```python
from build123d import *

# Parameters (mm, degrees)
CHAMFER1_SIZE                                  = 1.27
CBORE_FOR_2_SOCKET_HEAD_CAP_SCREW1_D           = 2.7051
CBORE_FOR_2_SOCKET_HEAD_CAP_SCREW1_DEPTH       = 12.7
CBORE_FOR_2_SOCKET_HEAD_CAP_SCREW1_CBORE_D     = 4.7625
CBORE_FOR_2_SOCKET_HEAD_CAP_SCREW1_CBORE_DEPTH = 2.1844
CUT_EXTRUDE1_DEPTH                             = 13.7
SKETCH7_R                                      = 1.27
CUT_EXTRUDE2_DEPTH                             = 13.7


with BuildPart() as part:
    # Sketch1 → Revolve1 (revolve)
    with BuildSketch(Plane.XY):
        Polygon((4, 19.05), (9.525, 19.05), (9.525, 12.7), (19.05, 12.7), (19.05, 0), (4, 0), align=None)
    revolve(axis=Axis((0, 24.600281955, 0), (0, -1, 0)))

    # Chamfer1
    chamfer1_edges = [part.edges().sort_by_distance(p)[0] for p in [
        (-19.05, 12.7, 0),
        (-9.525, 19.05, 0),
        (-4, 19.05, 0),
    ]]
    chamfer(chamfer1_edges, length=CHAMFER1_SIZE)

    # CBORE for #2 Socket Head Cap Screw1
    with Locations(Plane(origin=(0, 12.7, 0), x_dir=(1, 0, 0), z_dir=(0, 1, 0))):
        with Locations((-8.89, -8.89), (8.89, -8.89), (8.89, 8.89), (-8.89, 8.89)):
            CounterBoreHole(CBORE_FOR_2_SOCKET_HEAD_CAP_SCREW1_D / 2, CBORE_FOR_2_SOCKET_HEAD_CAP_SCREW1_CBORE_D / 2, CBORE_FOR_2_SOCKET_HEAD_CAP_SCREW1_CBORE_DEPTH, depth=CBORE_FOR_2_SOCKET_HEAD_CAP_SCREW1_DEPTH)

    # Sketch6 → Cut-Extrude1 (cut, through all)
    with BuildSketch(Plane(origin=(0, 12.7, 0), x_dir=(1, 0, 0), z_dir=(0, 1, 0))):
        with BuildLine():
            Line((12.999999, 1.8415), (18.960785262, 1.8415))
            ThreePointArc((18.960785262, 1.8415), (19.05, 0), (18.960785262, -1.8415))
            Line((18.960785262, -1.8415), (12.999999, -1.8415))
            ThreePointArc((12.999999, -1.8415), (9.9045, 0), (12.999999, 1.8415))
        make_face()
    extrude(amount=-CUT_EXTRUDE1_DEPTH, mode=Mode.SUBTRACT)

    # Sketch7 → Cut-Extrude2 (cut, through all)
    with BuildSketch(Plane(origin=(0, 12.7, 0), x_dir=(1, 0, 0), z_dir=(0, 1, 0))):
        with Locations((-12.7, 0)):
            Circle(SKETCH7_R)
    extrude(amount=-CUT_EXTRUDE2_DEPTH, mode=Mode.SUBTRACT)


solid = part.part
```
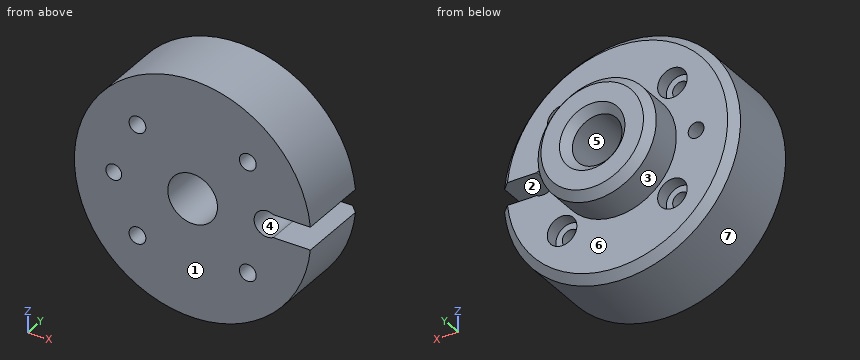
Geometry check sheet. Reference: the model listing, model coordinates, mm. Face numbers are marked on the shaded views. A direction names the side the tool comes from. Give positions to 0.01 mm unless a question says otherwise; leave off trailing zeros. Loops run counter-clockwise (first coordinate to the right, second up) from the corner with the lowest first, then second, coordinate; pieces in that order, holes last. Notation, with made-up numbers: M 66.5,62.5 L 81.5,62.5 A19 cw 81.5,81.5 Z; hole C 4,-11 d6. An arc over 180 degrees is marked long. Write item = value, one per line. Start each with the question number.
1. Section check A-A, the plane y = 6. Enter the section's corners in (x, z), plus the area to 3 significant figures.
2. Draft check along X on the marked faces 4, 5, 6 and 7. Enter one of: +X half, -X half, draft (parallel to the pull), parting line (faces both ways), or undercut.
3. Section check C-C, the plane z = 0. Give the number of separate pieces and of enclosed holes in the cut face, plus the area to 3 significant figures.
4. Section check D-D, the plane y = 16. Enter the section's corners in (x, z) (3 decimals).
5. Go/stop test with flat-tipped pins: P1, Ø4, axis at x = -7.5, y = 15.5, coming from the +Z side; P2, Ø10, axis at x = 14.5, z = -5, coming from the +Y side; P3, Ø2.5, axis at x = -8.89, z = -8.89, coming from the -Y side; P4, Ø6.5, axis at x = 15, y = 7, coming from the -Z side. Record where each tip stops, or that it passes through.
6. Thickness scan on probe 1 along X at (y, z) = (2.25, -8.89); probe 2 along X at (y, z) = (11.45, -8.89). Record the ranges inside material, lowest first.
7. Tool access check on the marked faces 1, 2 and 3. Record the directions out of +Z, -Z, +X, -X, +Y, -Y that give a thin tool (end or side, any length) a straight path to the whole face; none if there is none.
8. Section check B-B, the plane x = 0. Enter the section's corners in (y, z) (3 decimals).
Values follow:
q1.outline = M 13,-1.84 A2.1 cw long 13,1.84 L 18.96,1.84 A19.05 ccw long 18.96,-1.84 Z; hole C -12.7,0 d2.54; hole C -8.89,-8.89 d2.71; hole C -8.89,8.89 d2.71; hole C 0,0 d8; hole C 8.89,-8.89 d2.71; hole C 8.89,8.89 d2.71
q1.area = 1,030 mm^2
q2.face_4 = undercut
q2.face_5 = undercut
q2.face_6 = draft
q2.face_7 = parting line
q3.separate_pieces = 3
q3.enclosed_holes = 0
q3.area = 300 mm^2
q4.outline = C 0,0 d19.05; hole C 0,0 d8
q5.P1 = 7.78
q5.P2 = 12.7
q5.P3 = through
q5.P4 = -14.99
q6.probe_1 = -16.85 to -10.24, -7.54 to 7.54, 10.24 to 16.85
q6.probe_2 = -16.83 to -11.27, -6.51 to 6.51, 11.27 to 16.83
q7.face_1 = +Z, -Z, +X, -X, -Y
q7.face_2 = +X, +Y, -Y
q7.face_3 = +Y
q8.outline = M 0,-19.05 L 11.43,-19.05 L 12.7,-17.78 L 12.7,-9.525 L 17.78,-9.525 L 19.05,-8.255 L 19.05,-5.27 L 17.78,-4 L 0,-4 Z; M 0,4 L 17.78,4 L 19.05,5.27 L 19.05,8.255 L 17.78,9.525 L 12.7,9.525 L 12.7,17.78 L 11.43,19.05 L 0,19.05 Z
